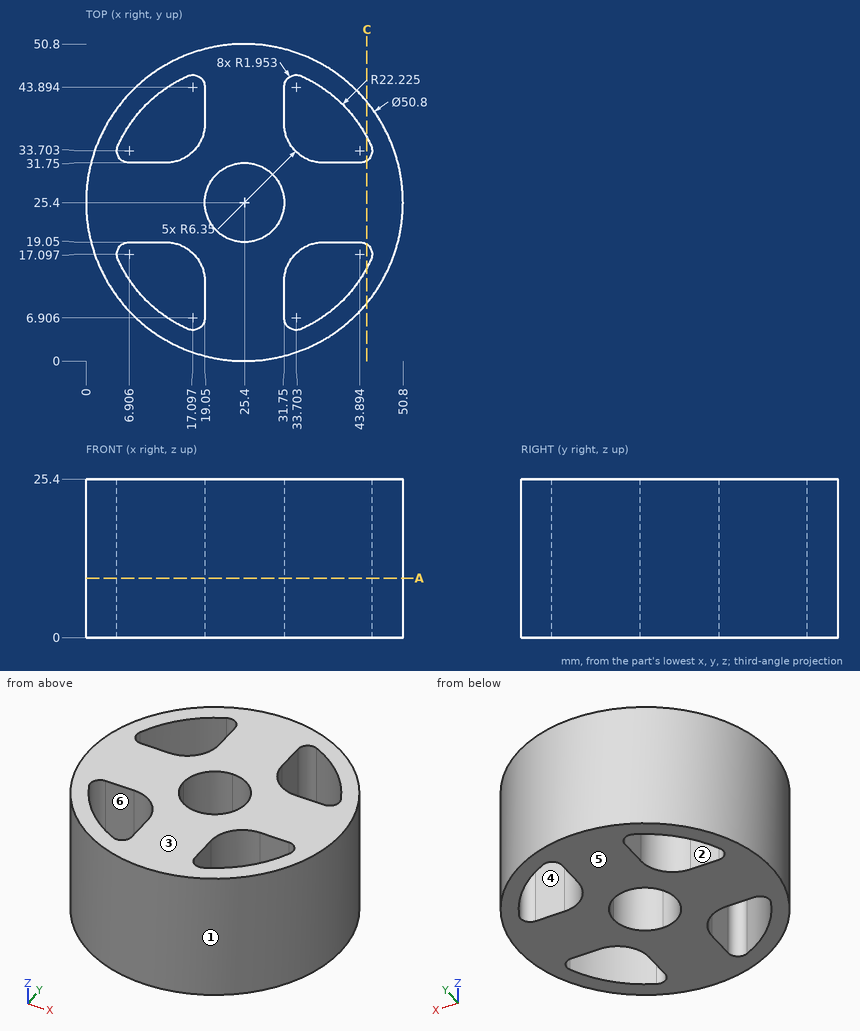
The figure shows three views and two pictorial views of one solid part (mm, origin at its lowest corner). Answer the questions. A direction names the side the tool comes from. Give positions to 0.01 mm unless a question says otherwise; leave off trailing zeros. Loops run counter-clockwise (first coordinate to the right, second up) from the corner with the lowest first, then second, coordinate; pieces in that order, holes last. Notation, with made-up numbers: (13, 14.5) -> (56, 14.5) arc R26 ccw to (56, 43.5) -> close; hole circle Ø10 at (76, 79.5). An arc over 180 degrees is marked (long way). Put each result on its own line as item: value. Start each with the question number.
Item 1: Each of these flat-tipped pins is pushed along its axis until it touches: P1, Ø12, axis at x = 37.5, z = 11.5, coming from the +Y side; P2, Ø1.7, axis at x = 10.5, z = 7.5, coming from the -Y side; P3, Ø4, axis at y = 33.5, z = 3.5, coming from the +X side; P4, Ø3, axis at x = 43, y = 16, coming from the +Z side. Where does it stop, or does it pass through?
Item 2: Which of the six approach directions +Z, -Z, +X, -X, +Y, -Y give full straight-line access (tool end or side, diameter ignored) to the marked faces 5 and 6?
Item 3: The part is cut by section C-C (x = 45). Give the vertices of the cut face in (y, z) (1 decimal).
Item 4: The part is cut by section A-A (z = 9.5). State how many separate pieces and enclosed holes the cut face has, then the cut area to 3 significant figures.
Item 5: The mould has two halves that part along X. Classify the marked faces 1, 2, 3 and 4: released by +X, released by -X, zero draft, split by the parting line, or undercut.
Item 6: Find the intervals of material crossed by L1, parallel to X at y = 39, z = 13.25; L2, parallel to Y at x = 25.5, z = 20; L3, parallel to Y at x = 16, z = 11.75 (1 decimal), in increasing order. Write a range as [from, to].
Answers below:
1. P1: y = 50.06
1. P2: y = 4.24
1. P3: x = 50.06
1. P4: through
2. face 5: -Z, +X, -X, +Y, -Y
2. face 6: +Z, -Z
3. outline: (9.2, 0) -> (14.9, 0) -> (14.9, 25.4) -> (9.2, 25.4) -> close; (18.7, 0) -> (32.1, 0) -> (32.1, 25.4) -> (18.7, 25.4) -> close; (35.9, 0) -> (41.6, 0) -> (41.6, 25.4) -> (35.9, 25.4) -> close
4. separate pieces: 1
4. enclosed holes: 5
4. area: 1,350 mm2
5. face 1: split by the parting line
5. face 2: undercut
5. face 3: zero draft
5. face 4: undercut
6. L1: [3.95, 7.82], [19.05, 31.75], [42.98, 46.85]
6. L2: [0, 19.05], [31.75, 50.8]
6. L3: [1.8, 5.3], [18.1, 32.7], [45.5, 49]
